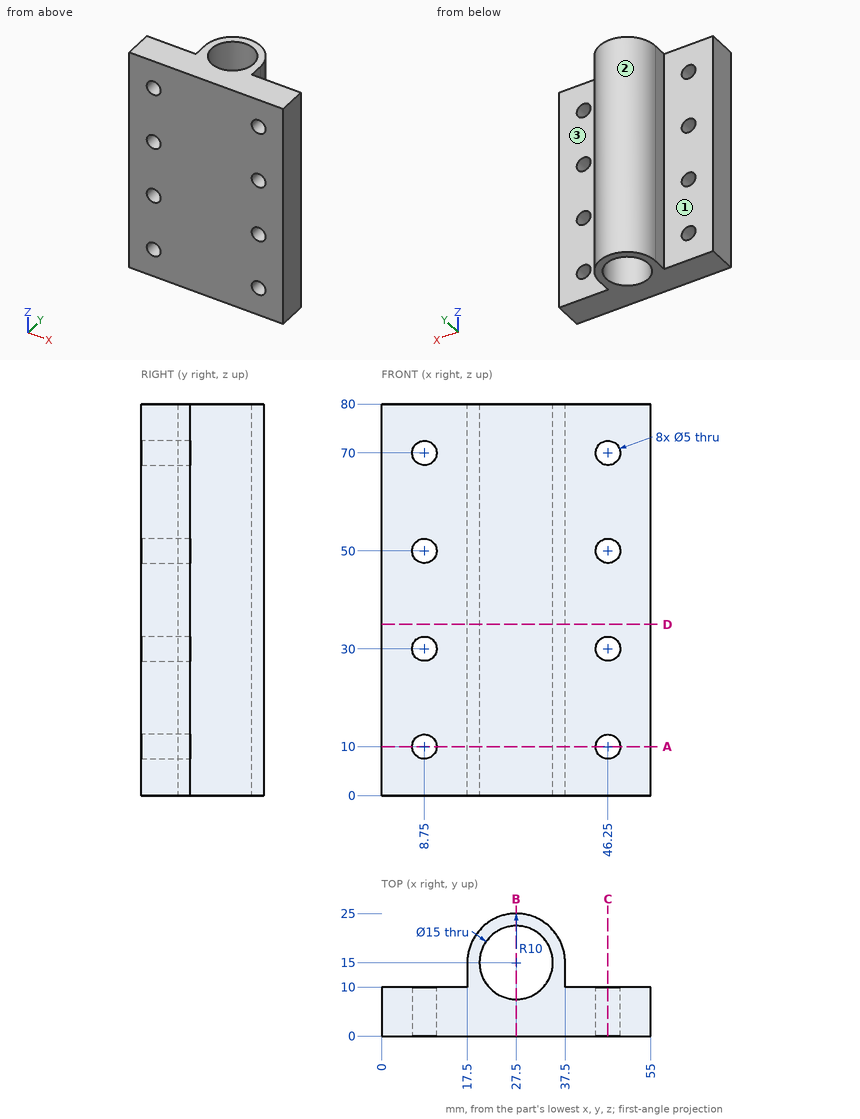
Design review of the part shown in the three views and the two pictorial views. Dimensions are in mm from the part's minimum x, y and z. A direction names the side the tool comes from. Round coordinates to 2 decimals unless told otherwise and drop trailing zeros. Loops run counter-clockwise (first coordinate to the right, second up) from the corner with the lowest first, then second, coordinate; pieces in that order, holes last.
1) Consider section A-A on z = 10. State the section outline as (x, y) points, then the cut area to 3 significant figures.
Values follow:
outline: (0, 0) - (6.25, 0) - (6.25, 10) - (0, 10) - close; (11.25, 0) - (43.75, 0) - (43.75, 10) - (37.5, 10) - (37.5, 15) arc R10 ccw to (17.5, 15) - (17.5, 10) - (11.25, 10) - close; (48.75, 0) - (55, 0) - (55, 10) - (48.75, 10) - close; hole circle Ø15 at (27.5, 15)
area: 530 mm2
2) Consider section C-C on x = 46.25. State the section outline as (y, z) points, then the cut area to 3 significant figures.
Values follow:
outline: (0, 0) - (10, 0) - (10, 7.5) - (0, 7.5) - close; (0, 12.5) - (10, 12.5) - (10, 27.5) - (0, 27.5) - close; (0, 32.5) - (10, 32.5) - (10, 47.5) - (0, 47.5) - close; (0, 52.5) - (10, 52.5) - (10, 67.5) - (0, 67.5) - close; (0, 72.5) - (10, 72.5) - (10, 80) - (0, 80) - close
area: 600 mm2
3) Tool access review of the marked faces 1, 2 and 3: name each direction out of +Z, -Z, +X, -X, +Y, -Y from which nothing blocks a thin tool from reaching the whole face with its end or side.
Values follow:
face 1: +Z, -Z, -X, +Y
face 2: +Z, -Z, +Y
face 3: +Z, -Z, +X, +Y
4) Clearance check with flat-ended pins moving along their axes: P1, Ø3, axis at x = 46.25, z = 30, coming from the -Y side; P2, Ø5, axis at x = 34.5, z = 61.5, coming from the +Y side; P3, Ø5, axis at x = 42.5, z = 35, coming from the +Y side; P4, Ø1.5, axis at y = 12.5, z = 48, coming from the +X side. State where each tip first meets the part, or that it passes through.
Values follow:
P1: passes through
P2: stops at y = 23.93
P3: stops at y = 10
P4: stops at x = 37.5
5) Wall thickness on line 1 along Z through (x, y) = (8.75, 3.25); line 2 along X through (y, z) = (15.5, 14); line 3 along Y through (x, z) = (5.5, 65): over which ranges is each line inside the solid? List them lowest first.
Values follow:
line 1: z = 0 to 7.5, 12.5 to 27.5, 32.5 to 47.5, 52.5 to 67.5, 72.5 to 80
line 2: x = 17.51 to 20.02, 34.98 to 37.49
line 3: y = 0 to 10
6) Consider section D-D on z = 35. State the section outline as (x, y) points, then the cut area to 3 significant figures.
Values follow:
outline: (0, 0) - (55, 0) - (55, 10) - (37.5, 10) - (37.5, 15) arc R10 ccw to (17.5, 15) - (17.5, 10) - (0, 10) - close; hole circle Ø15 at (27.5, 15)
area: 630 mm2
7) Consider section B-B on x = 27.5. State the section outline as (y, z) points, then the cut area to 3 significant figures.
Values follow:
outline: (0, 0) - (7.5, 0) - (7.5, 80) - (0, 80) - close; (22.5, 0) - (25, 0) - (25, 80) - (22.5, 80) - close
area: 800 mm2
